```python
from build123d import *

# Parameters (mm, degrees)
RESSALTO_EXTRUS_O1_DEPTH = 10
CORTE_EXTRUS_O1_REACH    = 40.81
ESBO_O2_R                = 2.5
CORTE_EXTRUS_O2_DEPTH    = 10
ESBO_O5_R                = 13
CORTE_EXTRUS_O3_DEPTH    = 8
ESBO_O6_R                = 9
CORTE_EXTRUS_O4_DEPTH    = 29.200177304
FILETE1_R                = 5
ESBO_O7_R                = 1.5
CORTE_EXTRUS_O5_DEPTH    = 10


with BuildPart() as part:
    # Esboço1 → Ressalto-extrusão1 (new body)
    with BuildSketch(Plane.XY):
        Polygon((-22.5, 15), (22.5, 15), (22.5, 5), (11.5, 5), (11.5, -5), (22.5, -5), (22.5, -15), (-22.5, -15), align=None)
    extrude(amount=RESSALTO_EXTRUS_O1_DEPTH)

    # Corte-extrusão1: up to this face of the body (flat: up to its plane)
    corte_extrus_o1_end = Plane(part.part.faces().sort_by_distance((0, 15, 5))[0])
    # Esboço2 → Corte-extrusão1 (cut, up to the picked face)
    with BuildSketch(Plane.XZ.offset(15), mode=Mode.PRIVATE) as corte_extrus_o1_sk1:
        with Locations(Location((17.5, 5, 0), (0, 0, 270))):
            Circle(ESBO_O2_R)
    corte_extrus_o1_tool1 = split(extrude(corte_extrus_o1_sk1.sketch, amount=-CORTE_EXTRUS_O1_REACH, mode=Mode.PRIVATE), bisect_by=corte_extrus_o1_end, keep=Keep.BOTH, mode=Mode.PRIVATE)
    add(corte_extrus_o1_tool1.solids().sort_by(Axis((17.5, -15, 5), (0, 1, 0)))[0], mode=Mode.SUBTRACT)

    # Esboço4 → Corte-extrusão2 (cut)
    with BuildSketch(Plane.XY.offset(10)):
        with BuildLine():
            Line((11.5, 5), (11.5, -5))
            ThreePointArc((11.5, -5), (9.428932188, 0), (11.5, 5))
        make_face()
    extrude(amount=-CORTE_EXTRUS_O2_DEPTH, mode=Mode.SUBTRACT)

    # Esboço5 → Corte-extrusão3 (cut)
    with BuildSketch(Plane.XY.offset(10)):
        with Locations((-7.5, 0)):
            Circle(ESBO_O5_R)
    extrude(amount=-CORTE_EXTRUS_O3_DEPTH, mode=Mode.SUBTRACT)

    # Esboço6 → Corte-extrusão4 (cut, through all)
    with BuildSketch(Plane.XY.offset(2)):
        with Locations((-7.5, 0)):
            Circle(ESBO_O6_R)
    extrude(amount=-CORTE_EXTRUS_O4_DEPTH, mode=Mode.SUBTRACT)

    # Filete1
    filete1_edges = [part.edges().sort_by_distance(p)[0] for p in [
        (22.5, 10, 0),
        (22.5, 10, 10),
        (22.5, -10, 0),
        (22.5, -10, 10),
    ]]
    fillet(filete1_edges, radius=FILETE1_R - 0.0001)  # a hair under: the kernel refuses the full size

    # Esboço7 → Corte-extrusão5 (cut)
    with BuildSketch(Plane.XY.offset(10)):
        with Locations((-19.5, -12)):
            Circle(ESBO_O7_R)
        with Locations(Location((-19.5, 12, 0), (0, 0, 180))):
            Circle(ESBO_O7_R)
        with Locations((4.5, 12)):
            Circle(ESBO_O7_R)
        with Locations(Location((4.5, -12, 0), (0, 0, 180))):
            Circle(ESBO_O7_R)
    extrude(amount=-CORTE_EXTRUS_O5_DEPTH, mode=Mode.SUBTRACT)


solid = part.part
```
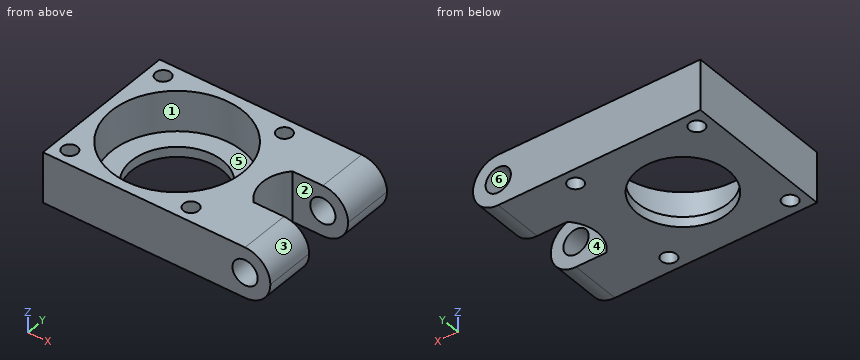
Verification items for the finished model (mm, model axes). Face numbers are marked on the shaded views. A direction names the side the tool comes from. Round coordinates to 2 decimals unless told otherwise and drop trailing zeros. Write each loop counter-clockwise with the first axis right and the second up, starting at its lowest first coordinate (ties: lowest second). Pieces come first, ordered by that corner, then holes.
1. Scan lines: L1, parallel to Y at x = 4.5, z = 7.25; L2, parallel to Y at x = 18, z = 8.5; L3, parallel to X at y = -11.5, z = 8. Record each from-to range of solid material in increasing order.
2. Section check C-C on x = -19.5. Enter the section's corners in (y, z).
3. Section check A-A on y = 0. Enter the section's corners in (x, z), plus the area to 3 significant figures.
4. Section check B-B on y = -12.5. State how many separate pieces and enclosed holes the cut face has, plus the area to 3 significant figures.
5. Access from +Z, -Z, +X, -X, +Y, -Y to the whole of each face (thin tool, end or side, straight path). Record for the marked faces 1, 2 and 3.
6. Draft check along Z on the marked faces 4, 5 and 6. Enter one of: +Z half, -Z half, draft (parallel to the pull), parting line (faces both ways), or undercut.
7. Gauge pin test, flat end, axial feed: P1, Ø3, axis at x = -9.5, y = -10.5, coming from the +Z side. Record the tip position at first contact, or that the pin passes through.
8. Section check D-D on z = 4. Enter the section's corners in (x, y).
Answer:
1. L1: y = -15 to -13.5, -10.5 to -5, 5 to 10.5, 13.5 to 15
1. L2: y = -15 to -5, 5 to 15
1. L3: x = -22.5 to -20.91, -18.09 to -13.56, -1.44 to 3.09, 5.91 to 21.5
2. outline: (-15, 0) - (-13.5, 0) - (-13.5, 10) - (-15, 10) - close; (-10.5, 0) - (10.5, 0) - (10.5, 10) - (5, 10) - (5, 2) - (-5, 2) - (-5, 10) - (-10.5, 10) - close; (13.5, 0) - (15, 0) - (15, 10) - (13.5, 10) - close
3. outline: (-22.5, 0) - (-16.5, 0) - (-16.5, 2) - (-20.5, 2) - (-20.5, 10) - (-22.5, 10) - close; (1.5, 0) - (9.43, 0) - (9.43, 10) - (5.5, 10) - (5.5, 2) - (1.5, 2) - close
3. area: 75.3 mm2
4. separate pieces: 3
4. enclosed holes: 1
4. area: 306 mm2
5. face 1: +Z
5. face 2: +Z, -Z, +X
5. face 3: +Z, +X, +Y, -Y
6. face 4: draft
6. face 5: +Z half
6. face 6: undercut
7. P1: stops at z = 2
8. outline: (-22.5, -15) - (15.21, -15) - (15.21, -5) - (11.5, -5) arc R7.07 cw to (11.5, 5) - (15.21, 5) - (15.21, 15) - (-22.5, 15) - close; (19.79, -15) - (22.4, -15) - (22.4, -5) - (19.79, -5) - close; (19.79, 5) - (22.4, 5) - (22.4, 15) - (19.79, 15) - close; hole circle Ø3 at (-19.5, -12); hole circle Ø3 at (-19.5, 12); hole circle Ø26 at (-7.5, 0); hole circle Ø3 at (4.5, -12); hole circle Ø3 at (4.5, 12)
